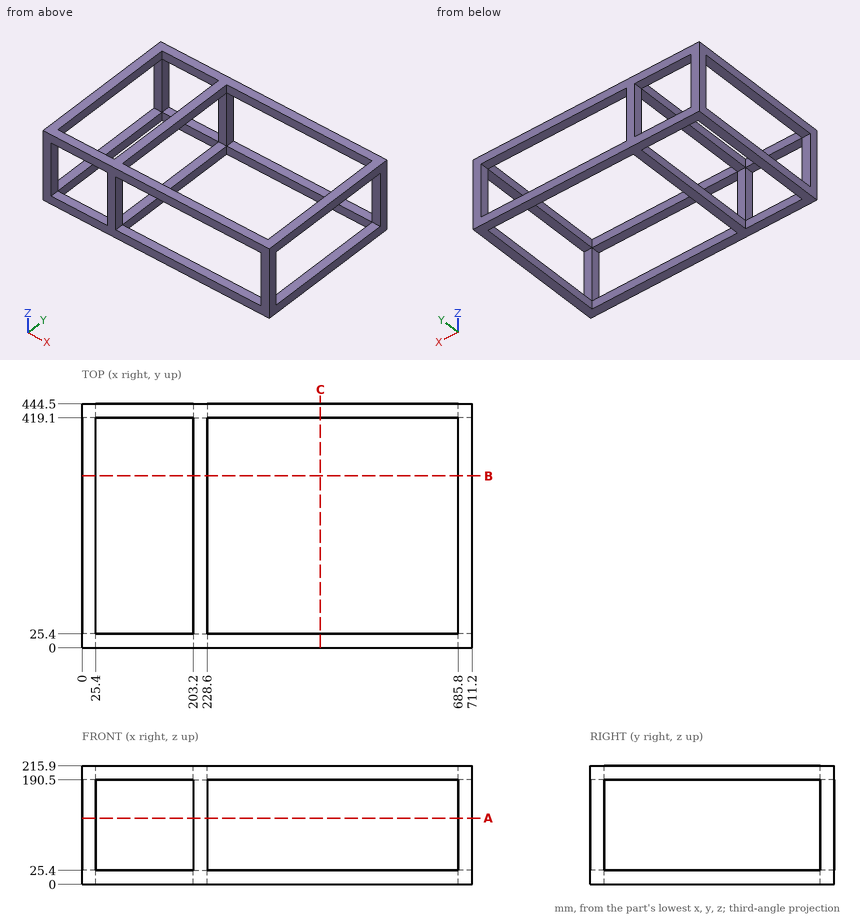
Drawing for the job (mm, zero at the part's lowest x, y, z). Give positions to 0.01 mm unless a question says otherwise; leave off trailing zeros. Loops run counter-clockwise (first coordinate to the right, second up) from the corner with the lowest first, then second, coordinate; pieces in that order, holes last.
(1) Band-saw the part on B-B (y = 313.5). Write the cut outline in (x, z).
Return value:
outline: (0, 0) - (25.4, 0) - (25.4, 25.4) - (0, 25.4) - close; (0, 190.5) - (25.4, 190.5) - (25.4, 215.9) - (0, 215.9) - close; (203.2, 0) - (228.6, 0) - (228.6, 25.4) - (203.2, 25.4) - close; (203.2, 190.5) - (228.6, 190.5) - (228.6, 215.9) - (203.2, 215.9) - close; (685.8, 0) - (711.2, 0) - (711.2, 25.4) - (685.8, 25.4) - close; (685.8, 190.5) - (711.2, 190.5) - (711.2, 215.9) - (685.8, 215.9) - close
(2) Drill centre lines: line 1 along X through (y, z) = (346, 12); line 2 along Y through (x, z) = (576.5, 205.5). Where is each one in solid material? Low to high.
Return value:
line 1: x = 0 to 25.4, 203.2 to 228.6, 685.8 to 711.2
line 2: y = 0 to 25.4, 419.1 to 444.5
(3) Band-saw the part on A-A (z = 120.5). Write the cut outline in (x, y).
Return value:
outline: (0, 0) - (25.4, 0) - (25.4, 25.4) - (0, 25.4) - close; (0, 419.1) - (25.4, 419.1) - (25.4, 444.5) - (0, 444.5) - close; (203.2, 0) - (228.6, 0) - (228.6, 25.4) - (203.2, 25.4) - close; (203.2, 419.1) - (228.6, 419.1) - (228.6, 444.5) - (203.2, 444.5) - close; (685.8, 0) - (711.2, 0) - (711.2, 25.4) - (685.8, 25.4) - close; (685.8, 419.1) - (711.2, 419.1) - (711.2, 444.5) - (685.8, 444.5) - close
(4) Band-saw the part on C-C (x = 434.5). Write the cut outline in (y, z).
Return value:
outline: (0, 0) - (25.4, 0) - (25.4, 25.4) - (0, 25.4) - close; (0, 190.5) - (25.4, 190.5) - (25.4, 215.9) - (0, 215.9) - close; (419.1, 0) - (444.5, 0) - (444.5, 25.4) - (419.1, 25.4) - close; (419.1, 190.5) - (444.5, 190.5) - (444.5, 215.9) - (419.1, 215.9) - close
